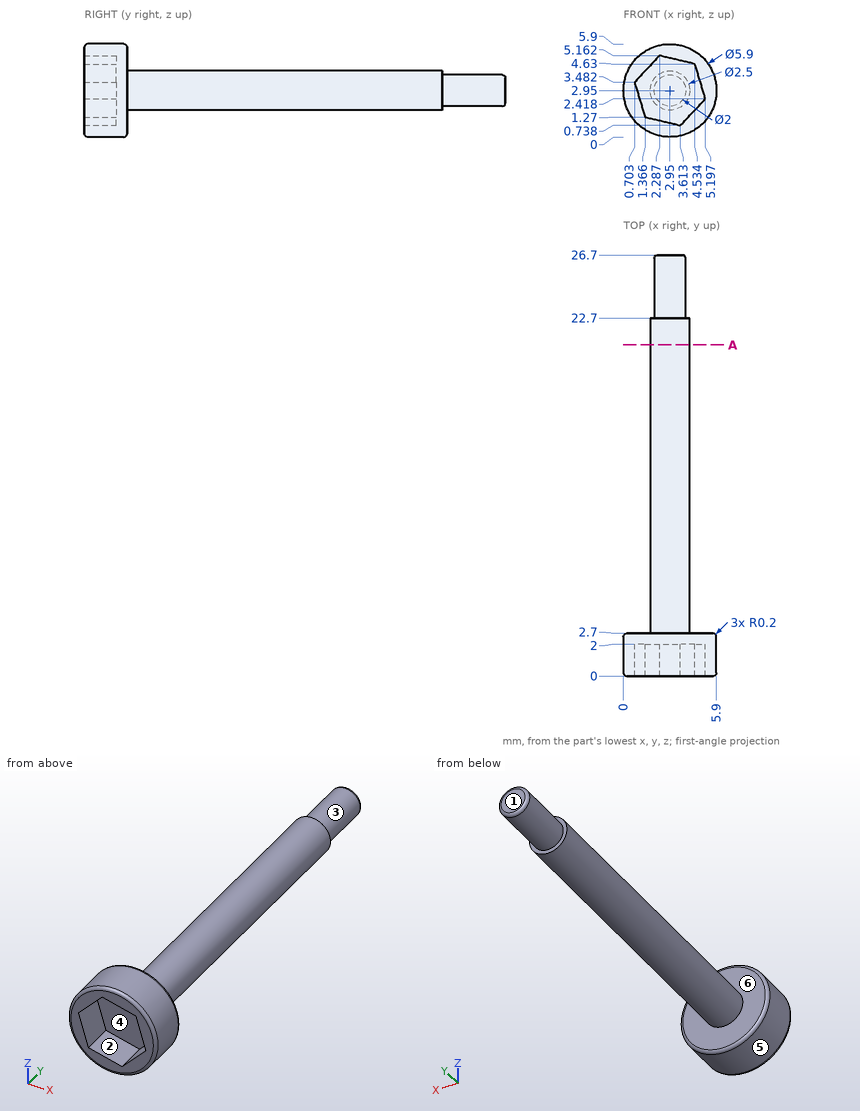
The drawing under review shows one solid part. Ordinate dimensions are in mm from its lowest x, y, z. A direction names the side the tool comes from. Coordinates: 2 decimals unless noted, no trailing zeros. Order: outer loops, then holes, each group sorted by start corner. A loop starts at its lowest first (then second) coordinate and runs counter-clockwise, first axis right, second up. Notation, with made-up numbers: (-34.75, 82.25) -> (-18.75, 82.25) arc R12 cw to (-18.75, 90.25) -> close; hole circle Ø8 at (-3, 12). An arc over 180 degrees is marked (long way). Use CSV: the item, a comma, the result in double quotes. Start each with the question number.
Item 1: We need section A-A, the plane y = 21. Give the boundary of the cut face in (x, z).
Item 2: Wall thickness on probe 1 along Y at (x, z) = (4.3, 2.8); probe 2 along Y at (x, z) = (2.3, 5.55); probe 3 along Z at (x, y) = (2.9, 7): over which ranges is each line inside the solid? List them lowest first.
Item 3: Draft analysis for pull direction X (two halves, no side actions). For the marked faces 1, 2 and 3, state which applies: pulls with the +X half, pulls with the -X half, needs draft (parallel to the pull), parting line crosses it, or undercut.
Item 4: For the marked faces 4, 5 and 6, list the 3-axis set-ups (+Z, -Z, +X, -X, +Y, -Y) from which the entire face can be reached by the end or side of a thin tool; tool diameter is ignored.
Item 5: Insertion check: pin 1 (1.3 mm diameter, centred on x = 3.5, z = 3.5, fed in from -Y); pin 2 (2 mm diameter, centred on y = 18, z = 5, fed in from +X); pin 3 (1 mm diameter, centred on x = 4, y = 9, fed in from +Z). Each pin has a flat end and moves straight along its axis. Give the tip position at first contact, or say it passes through.
Derived:
1,outline,"circle Ø2.5 at (2.95, 2.95)"
2,probe 1,"y = 2 to 2.7"
2,probe 2,"y = 0 to 2.7"
2,probe 3,"z = 1.7 to 4.2"
3,face 1,"needs draft"
3,face 2,"undercut"
3,face 3,"parting line crosses it"
4,face 4,"-Y"
4,face 5,"+Y, -Y"
4,face 6,"+Y"
5,pin 1,"stops at y = 2"
5,pin 2,"stops at x = 3.63"
5,pin 3,"stops at z = 4.07"
